Autodesk Inventor part; units mm, degrees
ref_plane "YZ Plane" through (0, 0, 0) normal (1, 0, 0) x (0, 1, 0)
ref_plane "XZ Plane" through (0, 0, 0) normal (0, 1, 0) x (-1, 0, 0)
ref_plane "XY Plane" through (0, 0, 0) normal (0, 0, 1) x (1, 0, 0)
sketch "Sketch1" plane through (0, 0, 0) normal (0, 1, 0) x (-1, 0, 0)
  line L0 (-3.175, 0) -> (-66.675, 0)
  line L1 (-69.85, -3.175) -> (-69.85, -213.3854)
  line L2 (-66.675, -216.5604) -> (-3.175, -216.5604)
  line L3 (0, -213.3854) -> (0, -3.175)
  arc A0 (0, -3.175) -> (-3.175, 0) centre (-3.175, -3.175) ccw
  arc A1 (-66.675, 0) -> (-69.85, -3.175) centre (-66.675, -3.175) ccw
  arc A2 (-69.85, -213.3854) -> (-66.675, -216.5604) centre (-66.675, -213.3854) ccw
  arc A3 (-3.175, -216.5604) -> (0, -213.3854) centre (-3.175, -213.3854) ccw
  line L4 (1.5875, -3.175) -> (1.5875, -213.3854)
  arc A4 (-3.175, -218.1479) -> (1.5875, -213.3854) centre (-3.175, -213.3854) ccw
  line L5 (-3.175, -218.1479) -> (-66.675, -218.1479)
  arc A5 (-71.4375, -213.3854) -> (-66.675, -218.1479) centre (-66.675, -213.3854) ccw
  line L6 (-71.4375, -213.3854) -> (-71.4375, -3.175)
  arc A6 (-66.675, 1.5875) -> (-71.4375, -3.175) centre (-66.675, -3.175) ccw
  line L7 (-66.675, 1.5875) -> (-3.175, 1.5875)
  arc A7 (1.5875, -3.175) -> (-3.175, 1.5875) centre (-3.175, -3.175) ccw
  point P0 (0, 0)
  point P1 (-69.85, -216.5604)
  point P2 (-69.85, 0)
  point P3 (0, -216.5604)
  dimension "d0" = 69.85
  dimension "d1" = 216.5604
  dimension "d2" = 3.175
extrude "Extrusion2" add sketch "Sketch1" along normal blind 3.175
sketch "Sketch4" plane through (3.175, 0, 1.5875) normal (0, 0, 1) x (1, 0, 0)
  circle A0 centre (31.75, 1.5875) radius 1.5875
  line L0 (0, 0) -> (0, 3.175)
  line L1 (0, 0) -> (63.5, 0)
  point P0 (-3.175, 0)
  dimension "d11" = 3.175
  dimension "d12" = 31.75
  dimension "d13" = 1.5875
extrude "Extrusion3" add sketch "Sketch4" along normal blind 2.54
sketch "Sketch5" plane through (66.675, 0, -218.1479) normal (0, 0, -1) x (-1, 0, 0)
  arc A0 (31.75, 0) -> (31.75, 3.175) centre (31.75, 1.5875) ccw
  circle A1 centre (31.75, 1.5875) radius 1.5875
  point P0 (66.675, 0)
  point P1 (31.75, 3.175)
  point P2 (31.75, 0)
extrude "Extrusion4" add sketch "Sketch5" along normal blind 2.54
properties part number "30t_8.5_in"
Read the model definition and answer for the solid it produces. Units are mm, in the model's axes. Coordinates: 2 decimals unless noted, no trailing zeros. Loops run counter-clockwise (first coordinate to the right, second up) from the corner with the lowest first, then second, coordinate; pieces in that order, holes last. Notation, with made-up numbers: (-31, 61) -> (-22, 61) arc R25 cw to (-22, 90) -> close; hole circle Ø1 at (55.25, -38.75). An arc over 180 degrees is marked (long way). Write item = value, one per line. Start each with the question number.
1) Given P1, Ø8, axis at x = 7, z = -26.5, coming from the -Y side; P2, Ø1.6, axis at x = 36.5, y = 1, coming from the +Z side; P3, Ø1, axis at x = 39, y = 1.5, coming from the +Z side; P4, Ø1.6, axis at x = 23, y = 2, coming from the -Z side, each flat-ended and moving along its own axis, determine where each tip first touches the part or whether it passes through.
2) The part is cut by section A-A, the plane x = 17. Determine the outline of the cut face in (y, z) (1 decimal), plus the area to 3 significant figures.
3) Find the intervals of material crossed by L1, parallel to X at y = 0.35, z = -72.5; L2, parallel to Z at x = 62, y = 1.1, in increasing order. Write a range as from..to.
Result:
q1.P1 = through
q1.P2 = 4.13
q1.P3 = 1.59
q1.P4 = -218.15
q2.outline = (0, -218.1) -> (3.2, -218.1) -> (3.2, -216.6) -> (0, -216.6) -> close; (0, 0) -> (3.2, 0) -> (3.2, 1.6) -> (0, 1.6) -> close
q2.area = 10.1 mm²
q3.L1 = -1.59..0, 69.85..71.44
q3.L2 = -218.15..-216.56, 0..1.59
